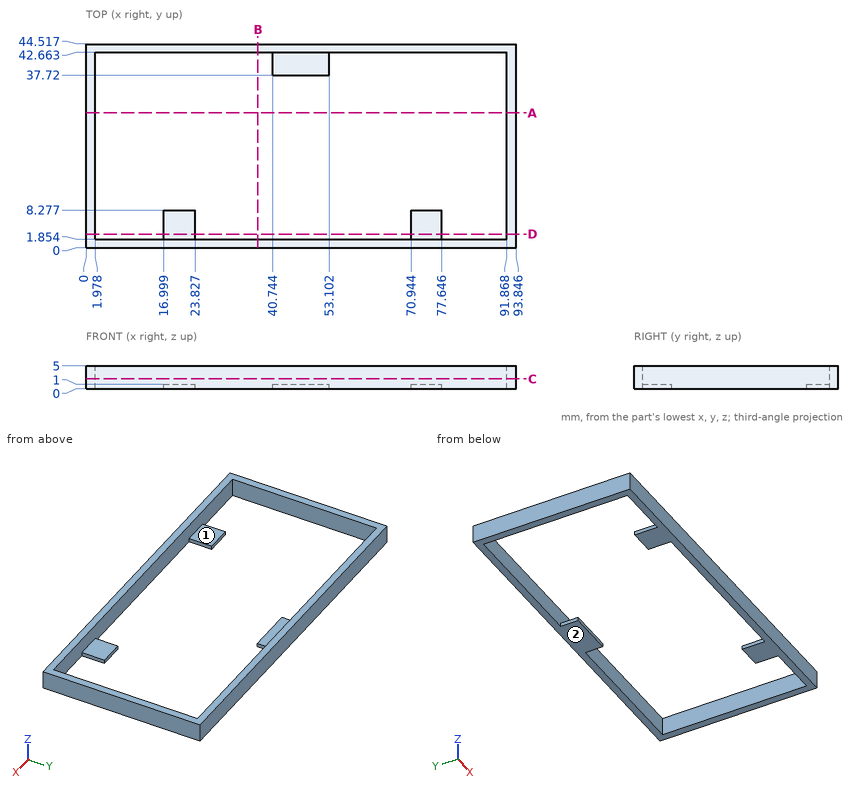
Drawing for the job (mm, zero at the part's lowest x, y, z). A direction names the side the tool comes from. Coordinates: 2 decimals unless noted, no trailing zeros. Order: outer loops, then holes, each group sorted by start corner. A loop starts at its lowest first (then second) coordinate and runs counter-clockwise, first axis right, second up. Notation, with made-up numbers: (88.25, 30) - (122.25, 30) arc R32 ccw to (122.25, 57) - close; hole circle Ø1 at (-0.5, 72.5). An arc over 180 degrees is marked (long way). Use a Markdown table: item, result. Add a question column.
(1) Which spindle directions (+Z, -Z, +X, -X, +Y, -Y) get a long thin tool onto all of the face, cutting with end or side? Do the marked faces 1 and 2. Say none if no direction does.
(2) Saw through at B-B (x = 37.5). Give the cut face in (y, z).
(3) Saw through at D-D (y = 3). Give the cut face in (x, z).
(4) Flat gauge pin, fed straight in: pin 1 (3 mm diameter, centred on x = 52, y = 37.5, fed in from +Z). Where does the tip first touch, or does it go through?
(5) Saw through at C-C (z = 2.2). Give the cut face in (x, y).
(6) Drill centre lines: line 1 along Y through (x, z) = (51, 3.55); line 2 along X through (y, z) = (35, 4.25); line 3 along Y through (x, z) = (46.5, 0.3). Where is each one in solid material? Low to high. Write a range as [from, to].
(7) Saw through at A-A (y = 29.5). Give the cut face in (x, z), then the cut area to 3 significant figures.
Solved:
| question | item | result |
|---|---|---|
| 1 | face 1 | +Z |
| 1 | face 2 | -Z, +X, -X, +Y, -Y |
| 2 | outline | (0, 0) - (1.85, 0) - (1.85, 5) - (0, 5) - close; (42.66, 0) - (44.52, 0) - (44.52, 5) - (42.66, 5) - close |
| 3 | outline | (0, 0) - (1.98, 0) - (1.98, 5) - (0, 5) - close; (17, 0) - (23.83, 0) - (23.83, 1) - (17, 1) - close; (70.94, 0) - (77.65, 0) - (77.65, 1) - (70.94, 1) - close; (91.87, 0) - (93.85, 0) - (93.85, 5) - (91.87, 5) - close |
| 4 | pin 1 | stops at z = 1 |
| 5 | outline | (0, 0) - (93.85, 0) - (93.85, 44.52) - (0, 44.52) - close; hole (1.98, 1.85) - (91.87, 1.85) - (91.87, 42.66) - (1.98, 42.66) - close |
| 6 | line 1 | y = [0, 1.85], [42.66, 44.52] |
| 6 | line 2 | x = [0, 1.98], [91.87, 93.85] |
| 6 | line 3 | y = [0, 1.85], [37.72, 44.52] |
| 7 | outline | (0, 0) - (1.98, 0) - (1.98, 5) - (0, 5) - close; (91.87, 0) - (93.85, 0) - (93.85, 5) - (91.87, 5) - close |
| 7 | area | 19.8 mm² |
